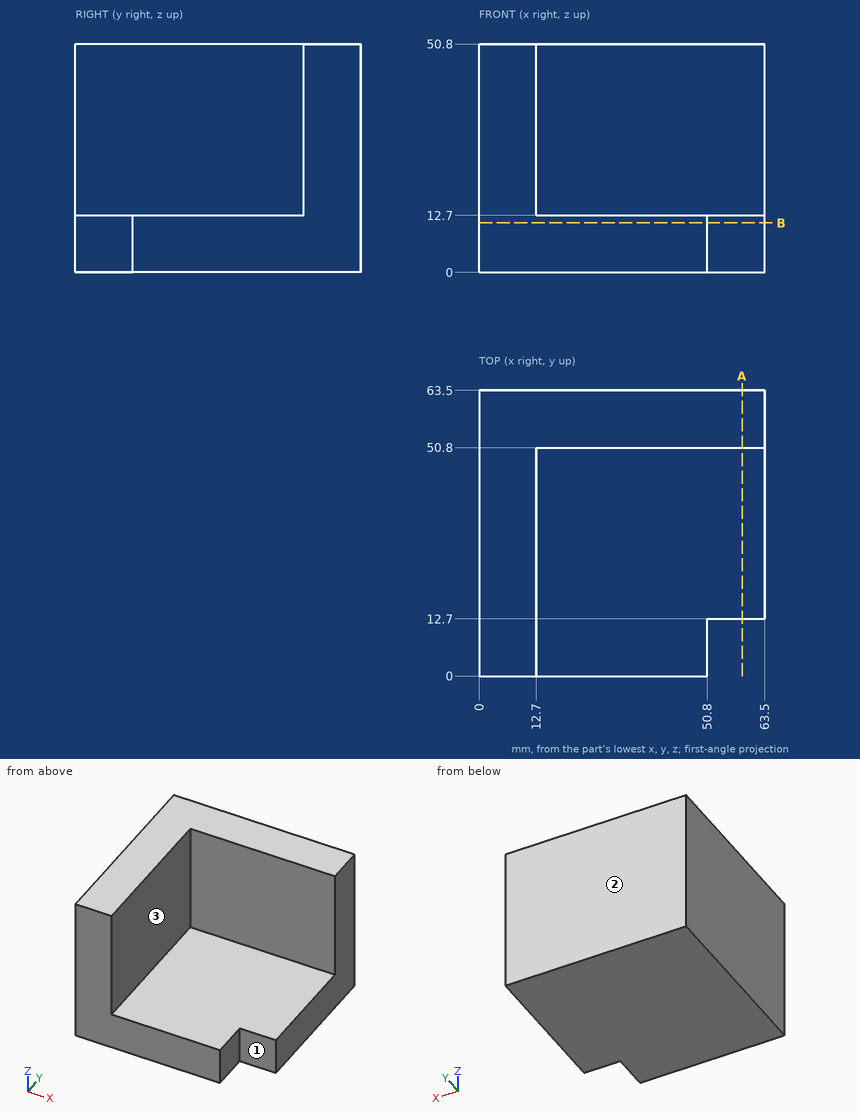
Study the drawing (mm; zero at the part's minimum x, y, z) and answer. A direction names the side the tool comes from. Coordinates: 2 decimals unless noted, no trailing zeros. Loops run counter-clockwise (first coordinate to the right, second up) from the corner with the lowest first, then second, coordinate; pieces in that order, holes last. Notation, with made-up numbers: M -21,23.25 L -8,23.25 A19 cw -8,31.25 Z; hole C 34.5,61 d1. An arc over 180 degrees is marked long. Answer as a JSON object with one key per item and string values. Group by question number.
Item 1: Consider L1, parallel to Y at x = 22, z = 48.5; L2, parallel to X at y = 20, z = 17. Determine where each line is inside the solid, lowest interval first.
Item 2: Section B-B (z = 11) is taken. Write down the section's boundary in (x, y).
Item 3: Section A-A (x = 58.5) is taken. Write down the section's boundary in (y, z), and give its area (3 significant figures).
Item 4: Each of these flat-tipped pins is pushed along its axis until it touches: P1, Ø6.5, axis at x = 55, z = 7.5, coming from the -Y side; P2, Ø6, axis at y = 56, z = 20, coming from the -X side; P3, Ø8, axis at y = 24, z = 33, coming from the +X side; P4, Ø10, axis at x = 26, y = 41, coming from the +Z side. Where does it stop, or does it pass through?
Item 5: Which of the six approach directions +Z, -Z, +X, -X, +Y, -Y give full straight-line access (tool end or side, diameter ignored) to the marked faces 1, 2 and 3?
Solved:
{
 "1": {"L1": "y = 50.8 to 63.5", "L2": "x = 0 to 12.7"},
 "2": {"outline": "M 0,0 L 50.8,0 L 50.8,12.7 L 63.5,12.7 L 63.5,63.5 L 0,63.5 Z"},
 "3": {"outline": "M 12.7,0 L 63.5,0 L 63.5,50.8 L 50.8,50.8 L 50.8,12.7 L 12.7,12.7 Z", "area": "1,130 mm2"},
 "4": {"P1": "stops at y = 12.7", "P2": "stops at x = 0", "P3": "stops at x = 12.7", "P4": "stops at z = 12.7"},
 "5": {"face 1": "+Z, -Z, +X, -Y", "face 2": "+Z, -Z, +X, -X, +Y", "face 3": "+Z, +X, -Y"}
}
